Study the drawing (mm; zero at the part's minimum x, y, z) and answer. A direction names the side the tool comes from. Round coordinates to 2 decimals unless told otherwise and drop trailing zeros. Order: outer loops, then holes, each group sorted by start corner. A loop starts at its lowest first (then second) coordinate and runs counter-clockwise, first axis right, second up. Notation, with made-up numbers: (13, 43.25) - (46, 43.25) arc R10 cw to (46, 51.25) - close; hole circle Ø11 at (88, 21). An arc over 180 degrees is marked (long way). Use one line per item in the form item = value. Start each with the question number.
Q1. For a pull along X with two mould halves and no side action, classify the marked faces 1, 2, 3 and 4 as +X half, -X half, draft (parallel to the pull), parting line (faces both ways), or undercut.
Q2. The part is cut by section B-B on x = 107.5. Determine the outline of the cut face in (y, z).
Q3. The part is cut by section A-A on y = 33. Determine the outline of the cut face in (x, z).
Q4. Find the intervals of material crossed by line 1 (X direction, y = 21.5, z = 57); line 2 (Z direction, x = 117, y = 46); line 3 (Y direction, x = 114, z = 80), in increasing order. Write a range as [from, to].
Q5. Which of the six approach directions +Z, -Z, +X, -X, +Y, -Y give full straight-line access (tool end or side, diameter ignored) to the marked faces 5, 6, 7, 8 and 9?
Q6. The part is cut by section D-D on y = 51. Determine the outline of the cut face in (x, z).
Q7. The part is cut by section C-C on z = 35.5. Determine the outline of the cut face in (x, y).
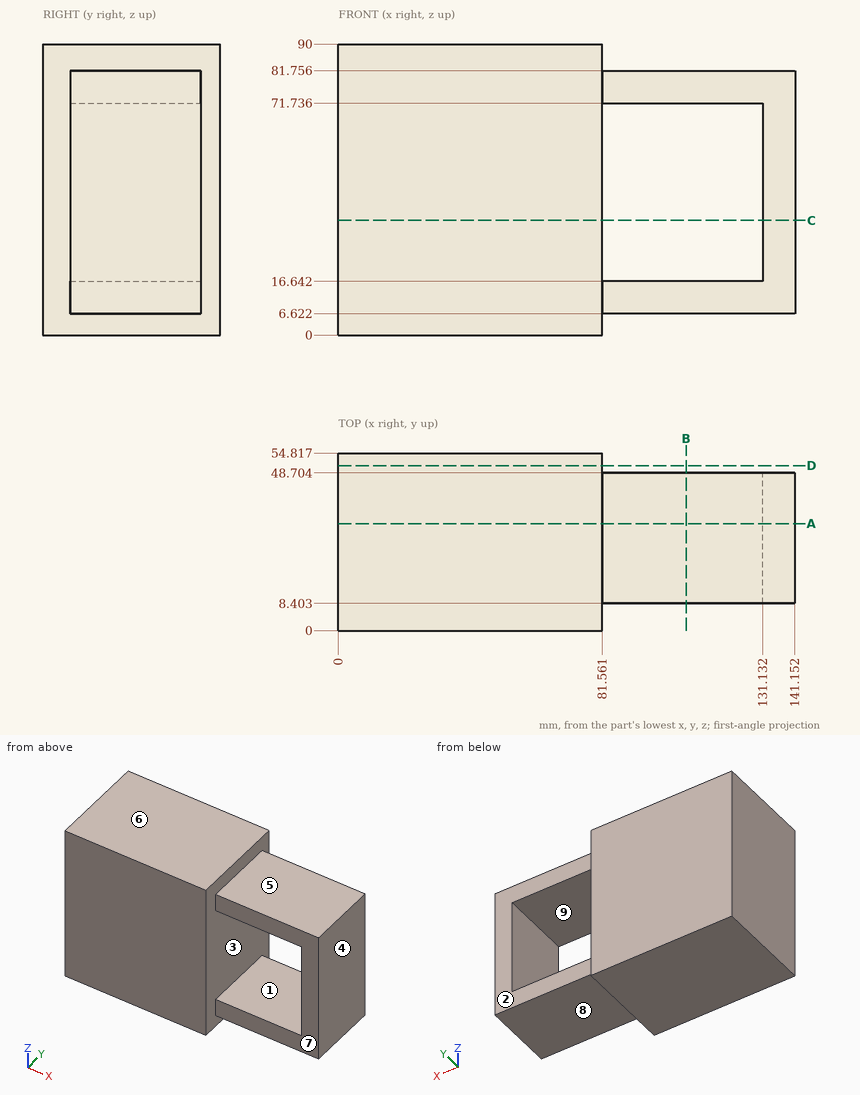
Found:
q1.face_1 = undercut
q1.face_2 = draft
q1.face_3 = undercut
q1.face_4 = +X half
q2.outline = (8.4, 6.62) - (48.7, 6.62) - (48.7, 16.64) - (8.4, 16.64) - close; (8.4, 71.74) - (48.7, 71.74) - (48.7, 81.76) - (8.4, 81.76) - close
q3.outline = (0, 0) - (81.56, 0) - (81.56, 6.62) - (141.15, 6.62) - (141.15, 81.76) - (81.56, 81.76) - (81.56, 90) - (0, 90) - close; hole (81.56, 16.64) - (131.13, 16.64) - (131.13, 71.74) - (81.56, 71.74) - close
q4.line_1 = [0, 81.56], [131.13, 141.15]
q4.line_2 = [6.62, 16.64], [71.74, 81.76]
q4.line_3 = [8.4, 48.7]
q5.face_5 = +Z, +X, +Y, -Y
q5.face_6 = +Z, +X, -X, +Y, -Y
q5.face_7 = +Z, -Z, +X, -Y
q5.face_8 = -Z, +X, +Y, -Y
q5.face_9 = +Y, -Y
q6.outline = (0, 0) - (81.56, 0) - (81.56, 90) - (0, 90) - close
q7.outline = (0, 0) - (81.56, 0) - (81.56, 54.82) - (0, 54.82) - close; (131.13, 8.4) - (141.15, 8.4) - (141.15, 48.7) - (131.13, 48.7) - close
